Can you work these out from the drawing? Everything is in mm from the part's minimum corner. A direction names the side the tool comes from. Coordinates: 2 decimals unless noted, no trailing zeros. Loops run counter-clockwise (first coordinate to the right, second up) from the corner with the lowest first, then second, coordinate; pieces in that order, holes last. Notation, with made-up numbers: M -36,80 L -10,80 A23 ccw -10,107 Z; hole C 37,21 d7. An arc over 180 degrees is marked long. Use CSV: the item, a comma, the result in double quotes. Start each with the question number.
Q1. If we section it at B-B (x = 65.5): Please give me the cut outline in (y, z), and give its area (3 significant figures).
Q2. For pin 1 Ø13 at (x, y) = (248.5, 17) entering from +Z; pin 2 Ø3 at (x, z) = (41, 29.5) entering from +Y, each with a flat end and sliding along its axis, tell me the tip position at first contact or that it passes through.
Q3. If we section it at A-A (y = 16.5): Please give me the cut outline in (x, z), and give its area (3 significant figures).
Q4. Which directions (+Z, -Z, +X, -X, +Y, -Y) give clear straight access to the entire face, cutting with the end or side of a thin tool? Please do the marked faces 1 and 2.
Q5. If we section it at C-C (z = 230.5): Please give me the cut outline in (x, y), and give its area (4 significant figures).
Q6. Please list where these lines run through material, in increasing order: probe 1 along X at (y, z) = (11.25, 5); probe 2 along Z at (x, y) = (380, 16); probe 3 along Y at (x, z) = (199, 153.5). Write a range as [from, to].
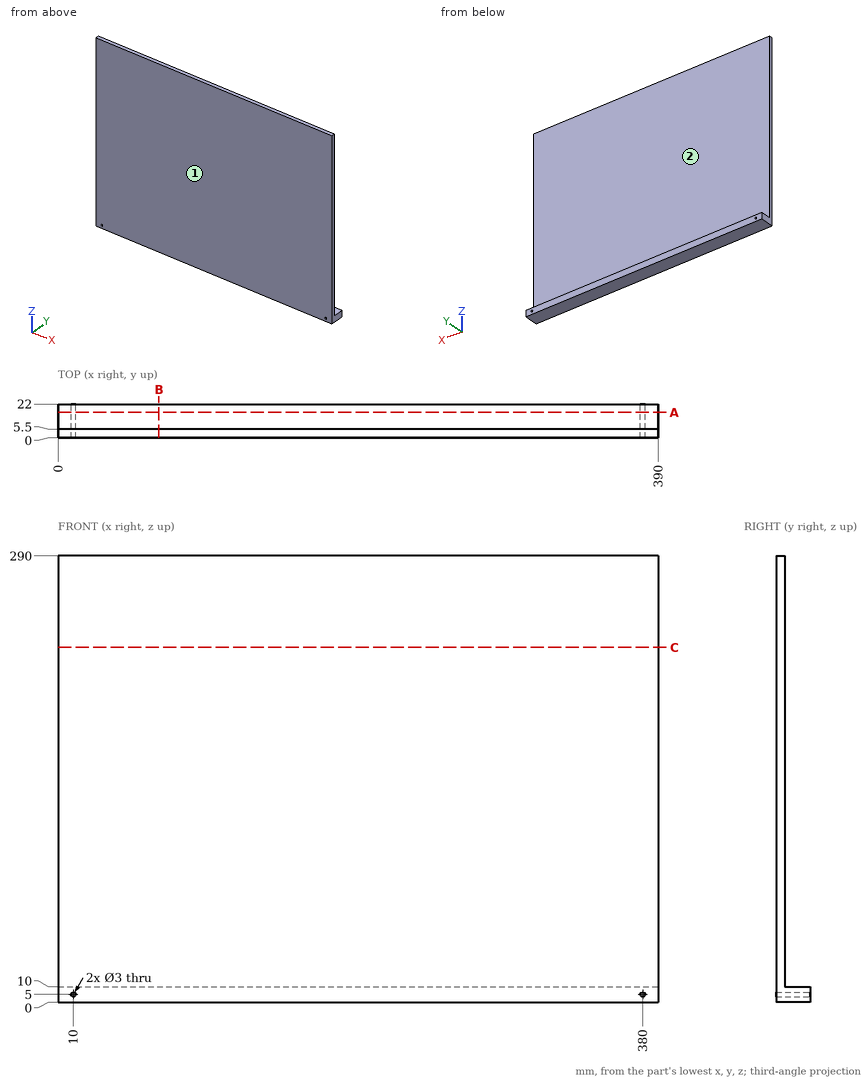
Results below:
1,outline,"M 0,0 L 22,0 L 22,10 L 5.5,10 L 5.5,290 L 0,290 Z"
1,area,"1,760 mm^2"
2,pin 1,"z = 10"
2,pin 2,"y = 5.5"
3,outline,"M 0,0 L 390,0 L 390,10 L 0,10 Z; hole C 10,5 d3; hole C 380,5 d3"
3,area,"3,890 mm^2"
4,face 1,"+Z, -Z, +X, -X, -Y"
4,face 2,"+Z, +X, -X, +Y"
5,outline,"M 0,0 L 390,0 L 390,5.5 L 0,5.5 Z"
5,area,"2,145 mm^2"
6,probe 1,"[0, 8.5], [11.5, 378.5], [381.5, 390]"
6,probe 2,"[0, 3.5], [6.5, 10]"
6,probe 3,"[0, 5.5]"
